The listing builds one solid part. Answer for the finished solid, in the listing's coordinates (mm). Face numbers are marked on the shaded views. A direction names the side the tool comes from. Coordinates: 2 decimals unless noted, no trailing zeros. Loops run counter-clockwise (first coordinate to the right, second up) from the corner with the lowest first, then second, coordinate; pieces in that order, holes last. Notation, with made-up numbers: (67, -19.5) -> (103, -19.5) arc R27 cw to (103, 10.5) -> close; hole circle Ø2 at (-26, 29). An arc over 180 degrees is marked (long way). Answer in a Markdown table with one row per item.
```python
from build123d import *

# Parameters (mm, degrees)
ESQUISSE1_R                  = 6.125
BOSS_EXTRU_1_DEPTH           = 20
ENL_V_MAT_EXTRU_1_DEPTH      = 31.16232128
ENL_V_MAT_EXTRU_1_DEPTH_BACK = 31.16232128
ESQUISSE2_R                  = 1.5


with BuildPart() as part:
    # Esquisse1 → Boss.-Extru.1 (new body)
    with BuildSketch(Plane.XY):
        with BuildLine():
            ThreePointArc((-9.023082899, -1.36), (0, -9.125), (9.023082899, -1.36))
            Line((9.023082899, -1.36), (19.125, -1.36))
            Line((19.125, -1.36), (19.125, 1.64))
            Line((19.125, 1.64), (9.125, 1.64))
            Line((9.125, 1.64), (9.125, 7.64))
            Line((9.125, 7.64), (19.125, 7.64))
            Line((19.125, 7.64), (19.125, 10.64))
            Line((19.125, 10.64), (-19.11513432, 10.64))
            Line((-19.11513432, 10.64), (-19.11513432, 7.64))
            Line((-19.11513432, 7.64), (-9.11513432, 7.64))
            Line((-9.11513432, 7.64), (-9.11513432, 1.64))
            Line((-9.11513432, 1.64), (-19.11513432, 1.64))
            Line((-19.11513432, 1.64), (-19.11513432, -1.36))
            Line((-19.11513432, -1.36), (-9.023082899, -1.36))
        make_face()
        Circle(ESQUISSE1_R, mode=Mode.SUBTRACT)
    extrude(amount=BOSS_EXTRU_1_DEPTH)

    # Esquisse2 → Enlèv. mat.-Extru.1 (cut, two sides: drawn at the far end of the back side and taken through both)
    with BuildSketch(Plane.XZ.offset(1.36).offset(-ENL_V_MAT_EXTRU_1_DEPTH_BACK)):
        with Locations(Location((-14.07013432, 10, 0), (0, 0, 180))):
            Circle(ESQUISSE2_R)
        with Locations(Location((14.08, 10, 0), (0, 0, 270))):
            Circle(ESQUISSE2_R)
    extrude(amount=ENL_V_MAT_EXTRU_1_DEPTH + ENL_V_MAT_EXTRU_1_DEPTH_BACK, mode=Mode.SUBTRACT)


solid = part.part
```
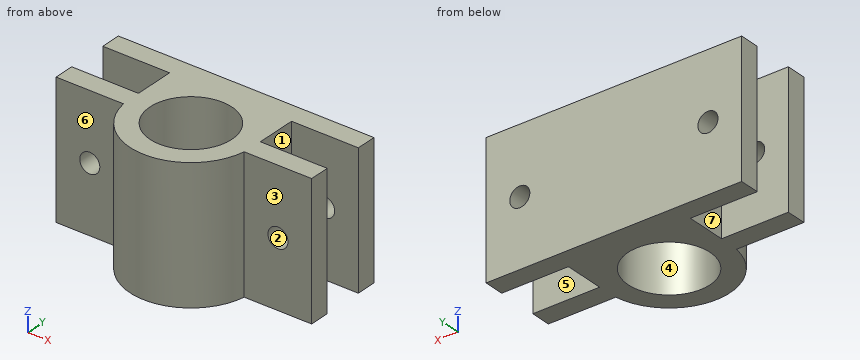
Item 1: A cutting plane is placed at A-A, the plane z = 10. Count the separate pieces of the cut face and the enclosed holes in it, plus the area to 3 significant figures.
Findings below:
| item | result |
|---|---|
| separate pieces | 5 |
| enclosed holes | 1 |
| area | 291 mm2 |
Item 2: A tool of negligible diameter and unlimited length cuts with its end or side. For the marked faces 5, 6 and 7, from which of +Z, -Z, +X, -X, +Y, -Y can it reach the whole face along a straight path? Write none if from no direction.
Findings below:
| item | result |
|---|---|
| face 5 | +Z, -Z, +X |
| face 6 | +Z, -Z, -X, -Y |
| face 7 | +Z, -Z, -X |
Item 3: Determine the mould class of the marked faces 1, 2, 3 and 4 for opening direction Y: +Y half, -Y half, draft (parallel to the pull), parting line (faces both ways), or undercut.
Findings below:
| item | result |
|---|---|
| face 1 | undercut |
| face 2 | draft |
| face 3 | -Y half |
| face 4 | undercut |
Item 4: A cutting plane is placed at C-C, the plane y = 0. Determine the outline of the cut face in (x, z) (3 decimals), plus the area to 3 significant figures.
Findings below:
| item | result |
|---|---|
| outline | (-19.115, 0) -> (-6.125, 0) -> (-6.125, 20) -> (-19.115, 20) -> close; (6.125, 0) -> (19.125, 0) -> (19.125, 20) -> (6.125, 20) -> close; hole circle Ø3 at (-14.07, 10); hole circle Ø3 at (14.08, 10) |
| area | 506 mm2 |
Item 5: Find the intervals of material crossed by probe 1 along Y at (x, z) = (13.5, 7); probe 2 along Z at (x, y) = (14.08, 9.5); probe 3 along X at (y, z) = (-0.5, 8.75) (3 decimals), in increasing order.
Findings below:
| item | result |
|---|---|
| probe 1 | y = -1.36 to 1.64, 7.64 to 10.64 |
| probe 2 | z = 0 to 8.5, 11.5 to 20 |
| probe 3 | x = -19.115 to -14.899, -13.241 to -6.105, 6.105 to 13.251, 14.909 to 19.125 |
Item 6: A cutting plane is placed at D-D, the plane x = 14.08. Determine the outline of the cut face in (y, z), plus the area to 3 significant figures.
Findings below:
| item | result |
|---|---|
| outline | (-1.36, 0) -> (1.64, 0) -> (1.64, 8.5) -> (-1.36, 8.5) -> close; (-1.36, 11.5) -> (1.64, 11.5) -> (1.64, 20) -> (-1.36, 20) -> close; (7.64, 0) -> (10.64, 0) -> (10.64, 8.5) -> (7.64, 8.5) -> close; (7.64, 11.5) -> (10.64, 11.5) -> (10.64, 20) -> (7.64, 20) -> close |
| area | 102 mm2 |
Item 7: A cutting plane is placed at B-B, the plane x = -12. Determine the outline of the cut face in (y, z), plus the area to 3 significant figures.
Findings below:
| item | result |
|---|---|
| outline | (-1.36, 0) -> (1.64, 0) -> (1.64, 20) -> (-1.36, 20) -> close; (7.64, 0) -> (10.64, 0) -> (10.64, 20) -> (7.64, 20) -> close |
| area | 120 mm2 |
Item 8: Flat-ended cylindrical pins translate along their axes: pin 1 Ø11 at (x, y) = (0, 0) entering from -Z; pin 2 Ø1.8 at (y, z) = (4, 11) entering from -X; pin 3 Ø3 at (y, z) = (4.5, 6) entering from +X (3 decimals); pin 4 Ø4 at (y, z) = (-3.5, 13) entering from -X. Find the tip coordinate at first contact, or state that the pin passes through.
Findings below:
| item | result |
|---|---|
| pin 1 | passes through |
| pin 2 | stops at x = -9.12 |
| pin 3 | stops at x = 9.125 |
| pin 4 | stops at x = -9 |
